Check sheet for the modelled part. Datum: model origin and axes. Units: mm. Give positions to 0.01 mm unless a question says otherwise; leave off trailing zeros. Write each loop counter-clockwise with the first axis right and the second up, starting at its lowest first coordinate (ties: lowest second). Pieces come first, ordered by that corner, then holes. Notation, with made-up numbers: (45, 6) -> (62, 6) arc R27 cw to (62, 39) -> close; hole circle Ø6 at (71.25, -16). An arc over 180 degrees is marked (long way). Write each question's results on one line, items separated by ' | '. Start each with the question number.
```python
from build123d import *

# Parameters (mm, degrees)
SKETCH1_W           = 127
SKETCH1_H           = 177.8
BOSS_EXTRUDE1_DEPTH = 25.4
CUT_EXTRUDE2_DEPTH  = 12.7


with BuildPart() as part:
    # Sketch1 → Boss-Extrude1 (new body)
    with BuildSketch(Plane(origin=(0, 0, 0), x_dir=(1, 0, 0), z_dir=(0, 1, 0))):
        Rectangle(SKETCH1_W, SKETCH1_H)
    extrude(amount=BOSS_EXTRUDE1_DEPTH)

    # Sketch2 → Cut-Extrude2 (cut)
    with BuildSketch(Plane(origin=(0, 25.4, 0), x_dir=(1, 0, 0), z_dir=(0, 1, 0))):
        Polygon((-57.15, 88.9), (57.15, 88.9), (44.45, -88.9), (-44.45, -88.9), align=None)
    extrude(amount=-CUT_EXTRUDE2_DEPTH, mode=Mode.SUBTRACT)


solid = part.part
```
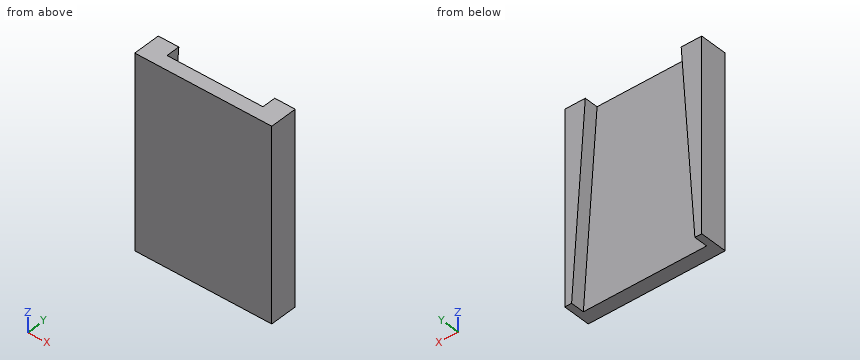
Item 1: Section check C-C on x = 47. Record the boundary of the cut face in (y, z), then the cut area to 3 significant figures.
Item 2: Section check D-D on z = -54. Record the boundary of the cut face in (x, y), then the cut area to 3 significant figures.
Item 3: Section check A-A on y = 19.5. Record the boundary of the cut face in (x, z).
Item 4: Thickness scan on probe 1 along Y at (x, z) = (-49.5, -59); probe 2 along X at (y, z) = (13.25, 21); probe 3 along X at (y, z) = (19.5, -62). Record the ranges inside material, lowest first. Write a range as from..to.
Item 5: Section check B-B on z = 38. Record the boundary of the cut face in (x, y), then the cut area to 3 significant figures.
Item 6: Depth check by flat-ended pin: pin 1 Ø2 at (x, z) = (-21.5, 36.5) entering from +Y. Enter the tip coordinate at first touch or a pass-through.
Check sheet entries:
1) outline: (0, -88.9) -> (12.7, -88.9) -> (12.7, 53.2) -> (25.4, 53.2) -> (25.4, 88.9) -> (0, 88.9) -> close | area: 2,710 mm^2
2) outline: (-63.5, 0) -> (63.5, 0) -> (63.5, 25.4) -> (54.66, 25.4) -> (54.66, 12.7) -> (-54.66, 12.7) -> (-54.66, 25.4) -> (-63.5, 25.4) -> close | area: 1,840 mm^2
3) outline: (-63.5, -88.9) -> (-57.15, -88.9) -> (-44.45, 88.9) -> (-63.5, 88.9) -> close; (44.45, 88.9) -> (57.15, -88.9) -> (63.5, -88.9) -> (63.5, 88.9) -> close
4) probe 1: y = 0..12.7 | probe 2: x = -63.5..-49.3, 49.3..63.5 | probe 3: x = -63.5..-55.23, 55.23..63.5
5) outline: (-63.5, 0) -> (63.5, 0) -> (63.5, 25.4) -> (48.09, 25.4) -> (48.09, 12.7) -> (-48.09, 12.7) -> (-48.09, 25.4) -> (-63.5, 25.4) -> close | area: 2,000 mm^2
6) pin 1: stops at y = 12.7
